```python
from build123d import *

# Parameters (mm, degrees)
SKETCH1_W           = 25.4
SKETCH1_H           = 25.4
SKETCH1_R           = 2.921
BOSS_EXTRUDE1_DEPTH = 3.81
FILLET1_R           = 2.54
SKETCH4_R           = 2.921
CUT_EXTRUDE1_DEPTH  = 40.757288755
FILLET2_R           = 2.54


with BuildPart() as part:
    # Sketch1 → Boss-Extrude1 (new body)
    with BuildSketch(Plane(origin=(0, 0, 0), x_dir=(1, 0, 0), z_dir=(0, 1, 0))):
        with Locations((12.7, 12.7)):
            Rectangle(SKETCH1_W, SKETCH1_H)
        with Locations(Location((12.7, 12.7, 0), (0, 0, 90))):
            Circle(SKETCH1_R, mode=Mode.SUBTRACT)
    extrude(amount=BOSS_EXTRUDE1_DEPTH)

    # Fillet1
    fillet1_edges = [part.edges().sort_by_distance(p)[0] for p in [
        (0, 1.905, -25.4),
        (25.4, 1.905, -25.4),
        (25.4, 1.905, 0),
        (0, 1.905, 0),
    ]]
    fillet(fillet1_edges, radius=FILLET1_R)

    # Sketch2 → Loft2 section 0
    with BuildSketch(Plane(origin=(0, 3.81, 0), x_dir=(1, 0, 0), z_dir=(0, 1, 0))):
        with BuildLine():
            Line((2.54, 25.4), (6.35, 25.4))
            Line((6.35, 25.4), (6.35, 0))
            Line((6.35, 0), (2.54, 0))
            Line((2.54, 0), (2.54, 25.4))
        make_face()
    # Sketch3 → Loft2 section 1
    with BuildSketch(Plane(origin=(0, 20.32, 0), x_dir=(1, 0, 0), z_dir=(0, 1, 0))):
        with BuildLine():
            Line((2.54, 19.05), (6.35, 19.05))
            Line((6.35, 19.05), (6.35, 6.35))
            Line((6.35, 6.35), (2.54, 6.35))
            Line((2.54, 6.35), (2.54, 19.05))
        make_face()
    loft()

    # Sketch2<3> → Loft3 section 0
    with BuildSketch(Plane(origin=(0, 3.81, 0), x_dir=(1, 0, 0), z_dir=(0, 1, 0))):
        with BuildLine():
            Line((22.86, 25.4), (19.05, 25.4))
            Line((19.05, 25.4), (19.05, 0))
            Line((19.05, 0), (22.86, 0))
            Line((22.86, 0), (22.86, 25.4))
        make_face()
    # Sketch3<3> → Loft3 section 1
    with BuildSketch(Plane(origin=(0, 20.32, 0), x_dir=(1, 0, 0), z_dir=(0, 1, 0))):
        with BuildLine():
            Line((19.05, 19.05), (22.86, 19.05))
            Line((22.86, 19.05), (22.86, 6.35))
            Line((22.86, 6.35), (19.05, 6.35))
            Line((19.05, 6.35), (19.05, 19.05))
        make_face()
    loft()

    # Sketch4 → Cut-Extrude1 (cut, through all)
    with BuildSketch(Plane.ZY.offset(-2.54)):
        with Locations(Location((-12.7, 15.24, 0), (0, 0, 270))):
            Circle(SKETCH4_R)
    extrude(amount=-CUT_EXTRUDE1_DEPTH, mode=Mode.SUBTRACT)

    # Fillet2
    fillet2_edges = [part.edges().sort_by_distance(p)[0] for p in [
        (20.955, 20.32, -6.35),
        (20.955, 20.32, -19.05),
        (4.445, 20.32, -19.05),
        (4.445, 20.32, -6.35),
    ]]
    fillet(fillet2_edges, radius=FILLET2_R)


solid = part.part
```
Here's how the part is built. I have some questions about the finished solid (model axes, mm). A direction names the side the tool comes from. Give positions to 0.01 mm unless a question says otherwise; leave off trailing zeros. Order: outer loops, then holes, each group sorted by start corner. A loop starts at its lowest first (then second) coordinate and runs counter-clockwise, first axis right, second up. Notation, with made-up numbers: (-0.5, 85) -> (55.5, 85) arc R30 ccw to (55.5, 123) -> close; hole circle Ø6 at (-20, 50.25). An arc over 180 degrees is marked (long way). Use CSV: the item, a comma, the result in double quotes. Start each with the question number.
Item 1: Thinking about a two-plate mould opening in Z: for faces 3 (the cylindrical face through (9.804, 1.878, -12.32)), 4 (the cylindrical face through (0.724, 1.932, -0.764)), 5 (the cylindrical face through (20.98, 19.86, -18.76)), which applies, pulls with the +Z half, pulls with the -Z half, needs draft (parallel to the pull), parting line crosses it, or undercut?
Item 2: Suppose I cut it at A-A (x = 12.7). List the corners of the cut face in (y, z) for me.
Item 3: If I drill on probe 1 along Y at (x, z) = (19.95, -12.7); probe 2 along Z at (x, y) = (12.7, 2.5); probe 3 along X at (y, z) = (2.5, -12.7), over which ranges is the centre line in solid material (lowest first)? Write a range as [from, to].
Item 4: On a 3-axis mill with a long thin cutter (end or side, diameter ignored), from which of +Z, -Z, +X, -X, +Y, -Y can I reach the whole of each face in a straight line? I mean faces 1 (the flat face through (1, 3.81, -13)), 2 (the flat face through (4.418, 11.355, -22.498)). Say none if no direction works.
Item 5: Suppose I cut it at B-B (x = 21.25). List the corners of the cut face in (y, z) for me.
Item 6: I'm going to push flat-ended pins straight in: P1, Ø1.5, axis at x = 22.5, y = 7.5, coming from the -Z side; P2, Ø3, axis at y = 17.5, z = -9.5, coming from the -X side; P3, Ø2, axis at x = 1, z = -7, coming from the +Y side; P4, Ø14, axis at x = 10.5, z = -18, coming from the +Y side. Where does each tip first touch, or does it pass through?
Item 7: Suppose I cut it at D-D (z = -12.7). Give the number of separate pieces and of enclosed holes in the cut face, and give its area (3 significant figures).
Item 8: Suppose I cut it at C-C (y = 1.5). List the corners of the cut face in (x, z) for me.
Answer block:
1,face 3,"undercut"
1,face 4,"pulls with the +Z half"
1,face 5,"pulls with the -Z half"
2,outline,"(0, -25.4) -> (3.81, -25.4) -> (3.81, -15.62) -> (0, -15.62) -> close; (0, -9.78) -> (3.81, -9.78) -> (3.81, 0) -> (0, 0) -> close"
3,probe 1,"y = [0, 12.32], [18.16, 20.32]"
3,probe 2,"z = [-25.4, -15.62], [-9.78, 0]"
3,probe 3,"x = [0, 9.78], [15.62, 25.4]"
4,face 1,"+Z, -Z, -X, +Y"
4,face 2,"-Z, +X, -X, +Y"
5,outline,"(0, -25.4) -> (3.81, -25.4) -> (18.69, -19.68) arc R2.54 ccw to (20.32, -17.31) -> (20.32, -8.09) arc R2.54 ccw to (18.69, -5.72) -> (3.81, 0) -> (0, 0) -> close; hole circle Ø5.84 at (15.24, -12.7)"
6,P1,"stops at z = -24.27"
6,P2,"stops at x = 2.54"
6,P3,"stops at y = 3.81"
6,P4,"stops at y = 20.32"
7,separate pieces,"4"
7,enclosed holes,"0"
7,area,"156 mm^2"
8,outline,"(0, -22.86) arc R2.54 ccw to (2.54, -25.4) -> (22.86, -25.4) arc R2.54 ccw to (25.4, -22.86) -> (25.4, -2.54) arc R2.54 ccw to (22.86, 0) -> (2.54, 0) arc R2.54 ccw to (0, -2.54) -> close; hole circle Ø5.84 at (12.7, -12.7)"
